Input: dimensioned drawing with shaded views. Units: mm. Origin: part minimum x, y, z. A direction names the side the tool comes from. Round coordinates to 2 decimals unless told otherwise and drop trailing zeros. Loops run counter-clockwise (first coordinate to the right, second up) from the corner with the lowest first, then second, coordinate; pieces in that order, holes last. Notation, with made-up numbers: (48.5, 89) - (103.5, 89) arc R7 ccw to (103.5, 97) - close; hole circle Ø2 at (15.5, 37). An arc over 180 degrees is marked (long way). One line per question, with ' | ' between items. Start each with the question number.
1. Cut plane D-D (z = 43). Return loops of the section in (x, y).
2. Pin query (flat end, axial travel): pin 1 (11 mm diameter, centred on x = 15, z = 86, fed in from +Y); pin 2 (3.5 mm diameter, centred on x = 23.5, y = 14, fed in from +Z); pin 3 (6 mm diameter, centred on x = 18, y = 27, fed in from -Z); pin 4 (8 mm diameter, centred on x = 9.5, y = 7, fed in from +Z) (1 decimal). Return the tip coordinate at first contact, or that it passes through.
3. Ray query, line 1 (Y direction, x = 27, z = 61.5); line 2 (X direction, y = 26, z = 86); line 3 (X direction, y = 22.5, z = 84.5) (1 decimal). Return the intervals inside material, ascending.
4. Cut plane A-A (z = 17). Return loops of the section in (x, y).
5. Cut plane B-B (x = 25). Return loops of the section in (y, z), then the cut area to 3 significant figures.
6. Mould query, pull axis Z, two halves, no side actions, for the marked faces 6, 7 and 8. Classes: pulls with the +Z half, pulls with the -Z half, needs draft (parallel to the pull), parting line crosses it, or undercut.
7. Access query for the marked faces 1, 2, 3, 4 and 5. Directions: +Z, -Z, +X, -X, +Y, -Y. A direction counts if a zero-diameter tool reaches every point of the face in a straight line with its end or side. Return the directions, or none.
8. Cut plane C-C (y = 23). Return loops of the section in (x, z), then the cut area to 3 significant figures.
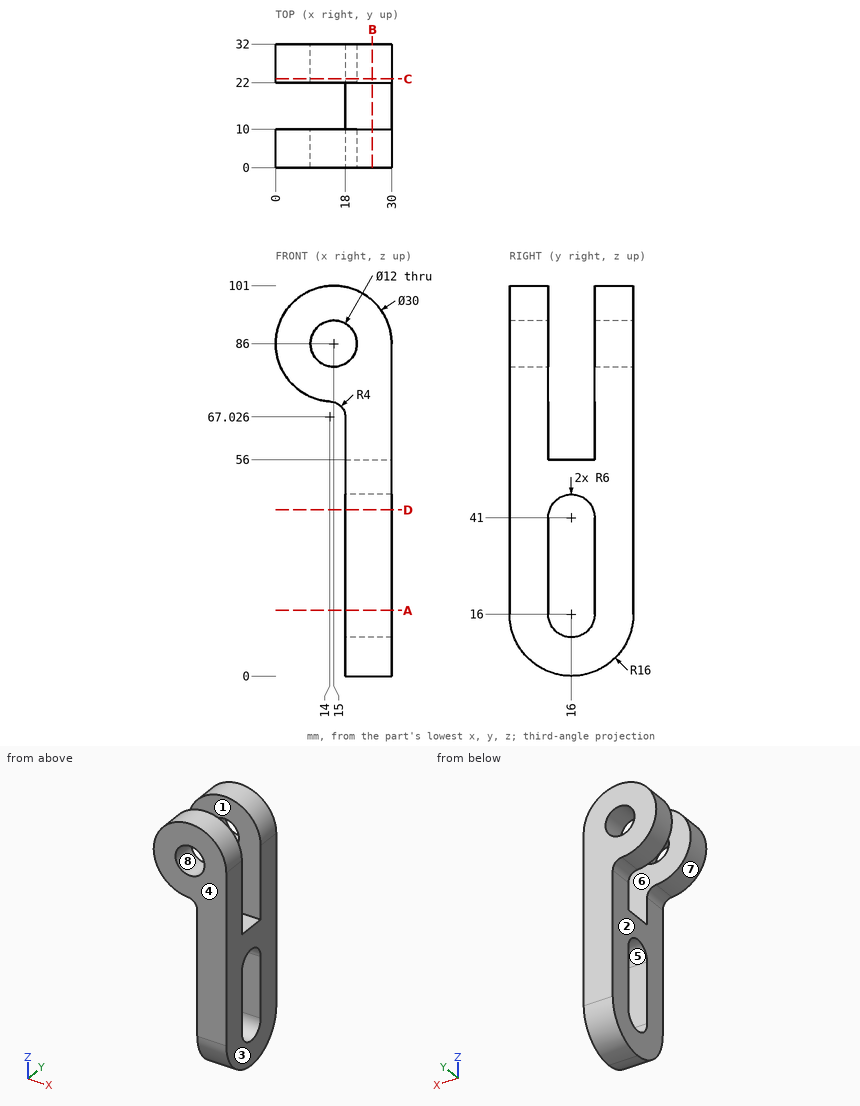
Answers follow:
1) outline: (18, 0) - (30, 0) - (30, 10.34) - (18, 10.34) - close; (18, 21.66) - (30, 21.66) - (30, 32) - (18, 32) - close
2) pin 1: passes through | pin 2: stops at z = 56 | pin 3: stops at z = 2.14 | pin 4: stops at z = 100.9
3) line 1: y = 0 to 10, 22 to 32 | line 2: x = 0 to 9, 21 to 30 | line 3: x = 0.1 to 9.2, 20.8 to 30
4) outline: (18, 0) - (30, 0) - (30, 10) - (18, 10) - close; (18, 22) - (30, 22) - (30, 32) - (18, 32) - close
5) outline: (0, 16) arc R16 ccw to (32, 16) - (32, 97.18) - (22, 97.18) - (22, 56) - (10, 56) - (10, 97.18) - (0, 97.18) - close; hole (10, 16) arc R6 ccw to (22, 16) - (22, 41) arc R6 ccw to (10, 41) - close | area: 2,090 mm2
6) face 6: needs draft | face 7: parting line crosses it | face 8: undercut
7) face 1: +Z, +X, -X | face 2: -Z, -X, +Y, -Y | face 3: +Z, -Z, +X, +Y, -Y | face 4: +Z, -Z, +X, -X, -Y | face 5: +X, -X
8) outline: (14.21, 71.02) arc R4 cw to (18, 67.03) - (18, 1.61) - (30, 1.61) - (30, 86) arc R15 ccw (long way) to start; hole circle Ø12 at (15, 86) | area: 1,480 mm2
